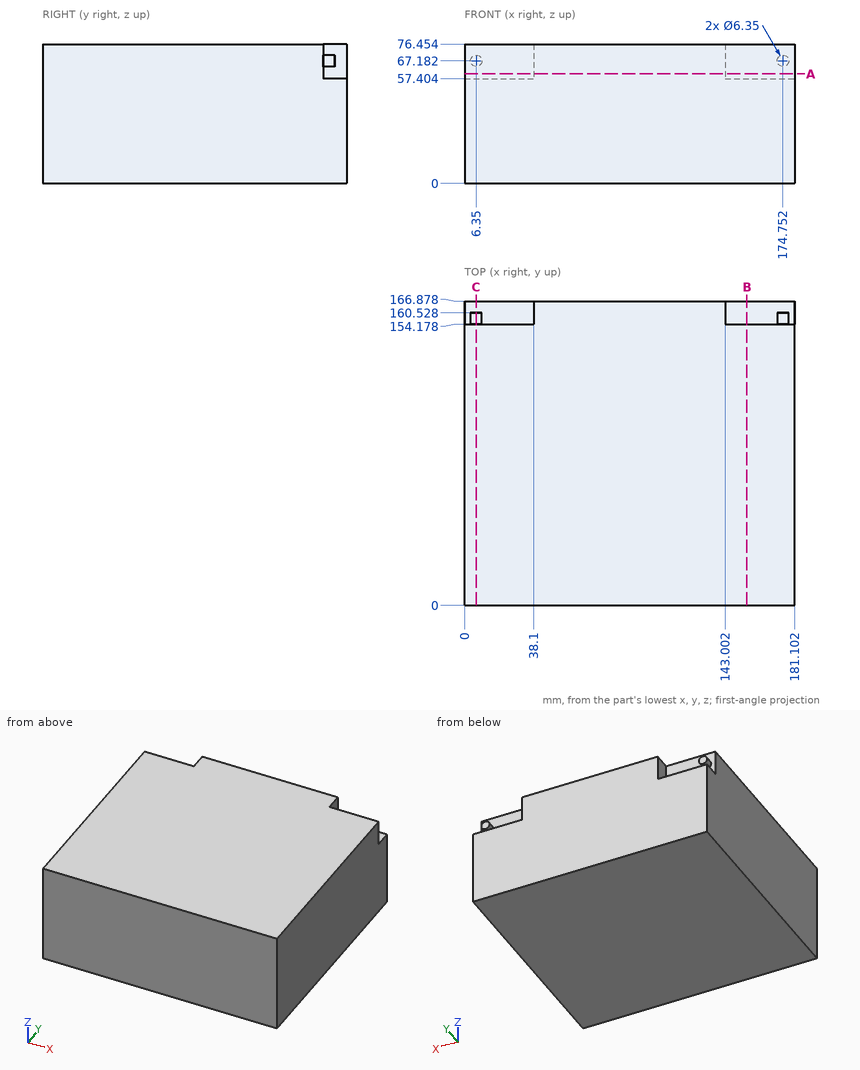
Geometry check sheet. Reference: drawing and pictorial views, mm from the part's lowest x, y, z. Give positions to 0.01 mm unless a question says otherwise; leave off trailing zeros. Write each loop counter-clockwise with the first axis right and the second up, starting at its lowest first coordinate (ties: lowest second). Pieces come first, ordered by that corner, then holes. Notation, with made-up numbers: M 57.25,19.5 L 101.25,19.5 A14 ccw 101.25,40.5 Z; hole C -11,-26.5 d7. An arc over 180 degrees is marked long. Put each result on its own line as item: value. Start each with the question number.
1. Section check A-A (z = 60). Record the cut outline in (x, y), and give its area (3 significant figures).
2. Go/stop test with flat-tipped pins: pin 1 Ø21 at (x, z) = (159.5, 62.5) entering from +Y; pin 2 Ø5.5 at (x, z) = (21.5, 67.5) entering from +Y; pin 3 Ø7 at (x, z) = (7.5, 66) entering from +Y; pin 4 Ø10 at (y, z) = (161, 66.5) entering from +X. Record where each tip stops, or that it passes through.
3. Section check C-C (x = 6.35). Record the cut outline in (y, z), and give its area (3 significant figures).
4. Section check B-B (x = 155). Record the cut outline in (y, z), and give its area (3 significant figures).
Answer list:
1. outline: M 0,0 L 181.1,0 L 181.1,154.18 L 143,154.18 L 143,166.88 L 38.1,166.88 L 38.1,154.18 L 0,154.18 Z
1. area: 29,300 mm2
2. pin 1: y = 166.88
2. pin 2: y = 154.18
2. pin 3: y = 160.53
2. pin 4: x = 177.93
3. outline: M 0,0 L 166.88,0 L 166.88,57.4 L 154.18,57.4 L 154.18,64.01 L 160.53,64.01 L 160.53,70.36 L 154.18,70.36 L 154.18,76.45 L 0,76.45 Z
3. area: 12,600 mm2
4. outline: M 0,0 L 166.88,0 L 166.88,57.4 L 154.18,57.4 L 154.18,76.45 L 0,76.45 Z
4. area: 12,500 mm2
